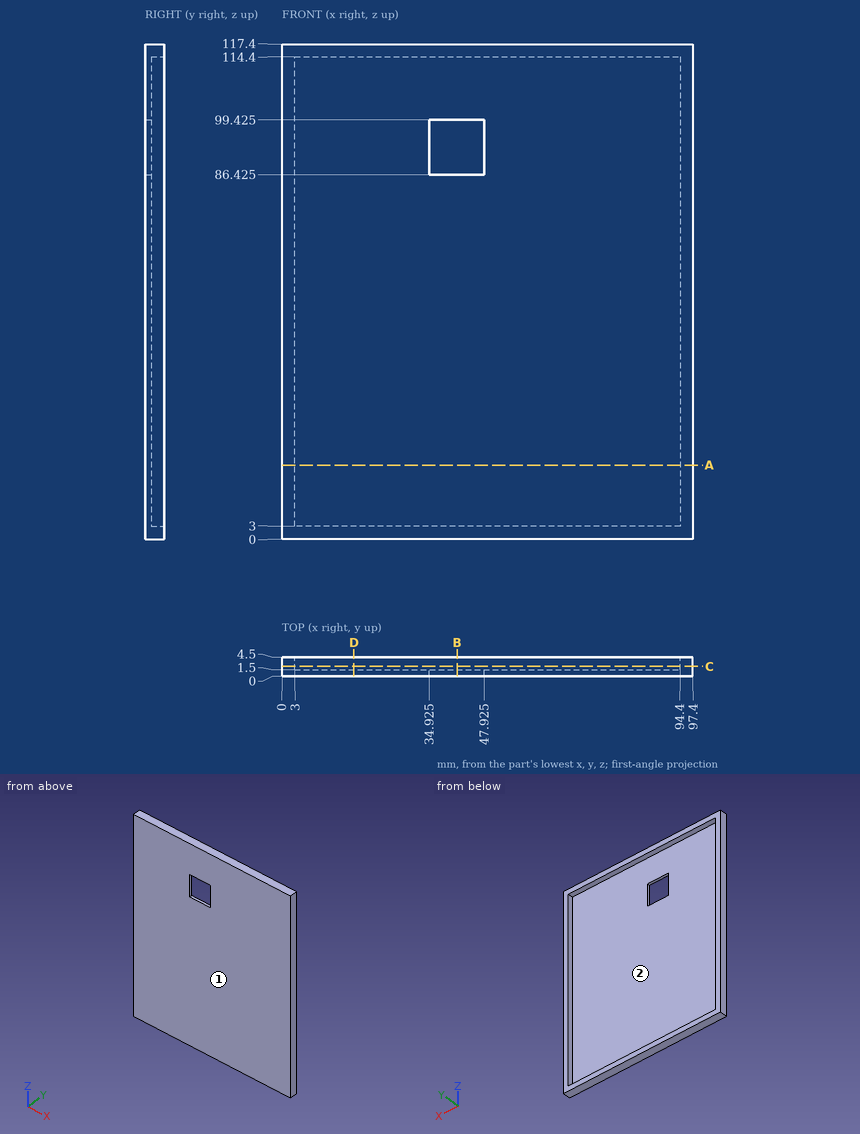
Design review of the part shown in the three views and the two pictorial views. Dimensions are in mm from the part's minimum x, y and z. Round coordinates to 2 decimals unless told otherwise and drop trailing zeros. Order: outer loops, then holes, each group sorted by start corner. A loop starts at its lowest first (then second) coordinate and runs counter-clockwise, first axis right, second up.
Item 1: Add section D-D, the plane x = 17. State the section outline as (y, z) points, and give its area (3 significant figures).
Working result:
outline: (0, 0) - (4.5, 0) - (4.5, 3) - (1.5, 3) - (1.5, 114.4) - (4.5, 114.4) - (4.5, 117.4) - (0, 117.4) - close
area: 194 mm2
Item 2: Add section A-A, the plane z = 17.5. State the section outline as (x, y) points.
Working result:
outline: (0, 0) - (97.4, 0) - (97.4, 4.5) - (94.4, 4.5) - (94.4, 1.5) - (3, 1.5) - (3, 4.5) - (0, 4.5) - close
Item 3: To check wall thickness, follow probe 1 along X at (y, z) = (2.95, 96.5); probe 2 along Z at (x, y) = (61, 3.1); probe 3 along Z at (x, y) = (40.5, 1.15) (3 decimals). State the ranges of each line that lie inside material, in increasing order.
Working result:
probe 1: x = 0 to 3, 94.4 to 97.4
probe 2: z = 0 to 3, 114.4 to 117.4
probe 3: z = 0 to 86.425, 99.425 to 117.4
Item 4: Add section B-B, the plane x = 41.5. State the section outline as (y, z) points (3 decimals).
Working result:
outline: (0, 0) - (4.5, 0) - (4.5, 3) - (1.5, 3) - (1.5, 86.425) - (0, 86.425) - close; (0, 99.425) - (1.5, 99.425) - (1.5, 114.4) - (4.5, 114.4) - (4.5, 117.4) - (0, 117.4) - close
Item 5: Add section C-C, the plane y = 2.3. State the section outline as (x, z) points.
Working result:
outline: (0, 0) - (97.4, 0) - (97.4, 117.4) - (0, 117.4) - close; hole (3, 3) - (94.4, 3) - (94.4, 114.4) - (3, 114.4) - close
Item 6: Draft analysis for pull direction X (two halves, no side actions). For the marked faces 1 and 2, state which applies: released by +X, released by -X, zero draft, split by the parting line, or undercut.
Working result:
face 1: zero draft
face 2: undercut
